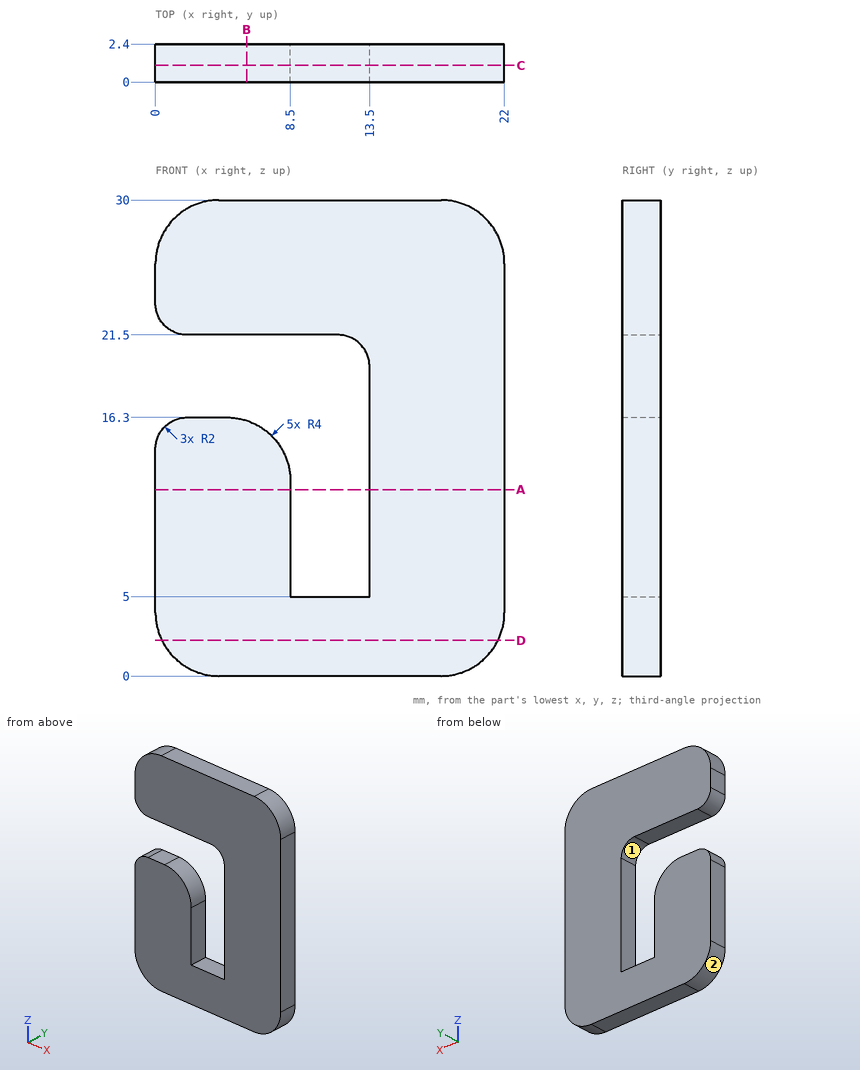
Could you check a few things on this drawing? It's one solid part, dimensions in mm from its lowest x, y, z. A direction names the side the tool comes from. Coordinates: 2 decimals unless noted, no trailing zeros. Order: outer loops, then holes, each group sorted by start corner. A loop starts at its lowest first (then second) coordinate and runs counter-clockwise, first axis right, second up.
1) Will these pins go through, and if not, where does the flat tip stop? pin 1 (0.7 mm diameter, centred on x = 7.5, y = 1, fed in from -Z); pin 2 (1.2 mm diameter, centred on x = 3, y = 1.5, fed in from +Z).
2) Imagine slicing it at B-B on x = 5.75. List the corners of the cut face in (y, z) for me.
3) I need wall thicknesses on line 1 (X direction, y = 1.25, z = 11); line 2 (Z direction, x = 10, y = 1.4); line 3 (Z direction, x = 2.25, y = 1.7). Which ranges of each line are inside material? Lowest first, please.
4) Imagine slicing it at A-A on z = 11.75. List the corners of the cut face in (x, y) for me, and give its area (3 significant figures).
5) Which directions (+Z, -Z, +X, -X, +Y, -Y) give clear straight access to the entire face, cutting with the end or side of a thin tool? Please do the marked faces 1 and 2.
6) Imagine slicing it at C-C on y = 1.05. List the corners of the cut face in (x, z) for me, and give its area (3 significant figures).
7) Imagine slicing it at D-D on z = 2.25. List the corners of the cut face in (x, y) for me.
Response values:
1. pin 1: stops at z = 0
1. pin 2: stops at z = 29.98
2. outline: (0, 0) - (2.4, 0) - (2.4, 16.1) - (0, 16.1) - close; (0, 21.5) - (2.4, 21.5) - (2.4, 30) - (0, 30) - close
3. line 1: x = 0 to 8.5, 13.5 to 22
3. line 2: z = 0 to 5, 21.5 to 30
3. line 3: z = 0.4 to 16.3, 21.5 to 29.6
4. outline: (0, 0) - (8.5, 0) - (8.5, 2.4) - (0, 2.4) - close; (13.5, 0) - (22, 0) - (22, 2.4) - (13.5, 2.4) - close
4. area: 40.8 mm2
5. face 1: -X, +Y, -Y
5. face 2: -Z, -X, +Y, -Y
6. outline: (0, 4) arc R4 ccw to (4, 0) - (18, 0) arc R4 ccw to (22, 4) - (22, 26) arc R4 ccw to (18, 30) - (4, 30) arc R4 ccw to (0, 26) - (0, 23.5) arc R2 ccw to (2, 21.5) - (11.5, 21.5) arc R2 cw to (13.5, 19.5) - (13.5, 5) - (8.5, 5) - (8.5, 12.3) arc R4 ccw to (4.5, 16.3) - (2, 16.3) arc R2 ccw to (0, 14.3) - close
6. area: 515 mm2
7. outline: (0.4, 0) - (21.6, 0) - (21.6, 2.4) - (0.4, 2.4) - close
